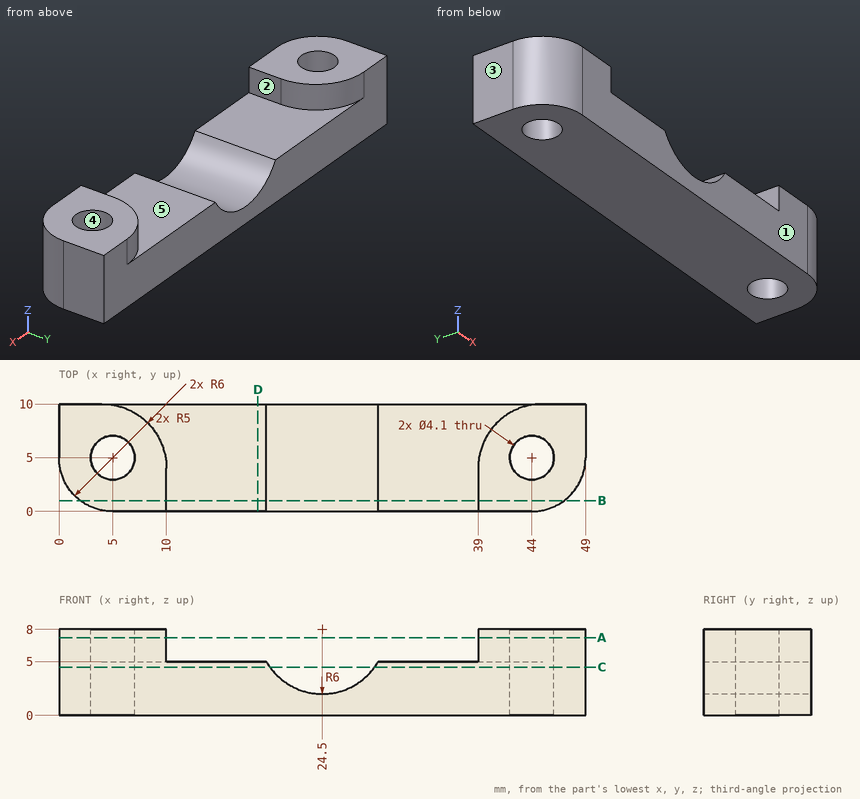
For this review, use the dimensioned drawing (mm, ordinates from the lowest corner) and the shaded views. A direction names the side the tool comes from. Round coordinates to 2 decimals unless told otherwise and drop trailing zeros. Loops run counter-clockwise (first coordinate to the right, second up) from the corner with the lowest first, then second, coordinate; pieces in that order, holes last. Notation, with made-up numbers: M -17.5,80.5 L 21.5,80.5 A18 cw 21.5,115.5 Z; hole C 39.25,-10.5 d4. An arc over 180 degrees is marked long. Answer as CSV lines item,"result".
1. We need section D-D (x = 18.5). Give the boundary of the cut face in (y, z), plus the area to 3 significant figures.
Outcome:
outline,"M 0,0 L 10,0 L 10,5 L 0,5 Z"
area,"50.0 mm2"
2. For the marked faces 4 and 5, list the 3-axis set-ups (+Z, -Z, +X, -X, +Y, -Y) from which the entire face can be reached by the end or side of a thin tool; tool diameter is ignored.
Outcome:
face 4,"+Z, -Z"
face 5,"+Z, +Y"
3. We need section A-A (z = 7.25). Give the boundary of the cut face in (x, y), plus the area to 3 significant figures.
Outcome:
outline,"M 0,5 A5 ccw 5,0 L 10,0 L 10,4 A6 ccw 4,10 L 0,10 Z; M 39,0 L 44,0 A5 ccw 49,5 L 49,10 L 45,10 A6 ccw 39,4 Z; hole C 5,5 d4.1; hole C 44,5 d4.1"
area,"147 mm2"
4. To check wall thickness, follow L1, parallel to Y at x = 5, z = 3.75; L2, parallel to X at y = 6.25, z = 5.75; L3, parallel to X at y = 5, z = 2.5. State the ranges of each line that lie inside material, in increasing order. Write a range as [from, to].
Outcome:
L1,"y = [0, 2.95], [7.05, 10]"
L2,"x = [0, 3.38], [6.62, 9.56], [39.44, 42.38], [45.62, 49]"
L3,"x = [0, 2.95], [7.05, 22.1], [26.9, 41.95], [46.05, 49]"
5. We need section C-C (z = 4.5). Give the boundary of the cut face in (x, y), plus the area to 3 significant figures.
Outcome:
outline,"M 0,5 A5 ccw 5,0 L 19.63,0 L 19.63,10 L 0,10 Z; M 29.37,0 L 44,0 A5 ccw 49,5 L 49,10 L 29.37,10 Z; hole C 5,5 d4.1; hole C 44,5 d4.1"
area,"355 mm2"
6. We need section B-B (y = 1). Give the boundary of the cut face in (x, z).
Outcome:
outline,"M 2,0 L 47,0 L 47,8 L 39,8 L 39,5 L 29.7,5 A6 cw 19.3,5 L 10,5 L 10,8 L 2,8 Z"
7. Draft analysis for pull direction X (two halves, no side actions). For the marked faces 1, 2 and 3, state which applies: pulls with the +X half, pulls with the -X half, needs draft (parallel to the pull), parting line crosses it, or undercut.
Outcome:
face 1,"needs draft"
face 2,"undercut"
face 3,"pulls with the -X half"
8. Insertion check: pin 1 Ø0.9 at (y, z) = (3, 7) entering from -X; pin 2 Ø3.5 at (y, z) = (2.5, 7) entering from +X. Each pin has a flat end and moves straight along its axis. Give the tip position at first contact, or say it passes through.
Outcome:
pin 1,"stops at x = 0.25"
pin 2,"stops at x = 48.94"
